Here's how the part is built. I have some questions about the finished solid (model axes, mm). Face numbers are marked on the shaded views. A direction names the side the tool comes from. Coordinates: 2 decimals unless noted, no trailing zeros. Write each loop counter-clockwise with the first axis right and the second up, starting at its lowest first coordinate (ties: lowest second). Pieces come first, ordered by that corner, then holes. Notation, with made-up numbers: (35, 42.5) - (67, 42.5) arc R13 ccw to (67, 65.5) - close; hole circle Ø10 at (20, 50). An arc over 180 degrees is marked (long way). Answer in a Markdown table with one row per item. Add a question column.
Item 1: Imagine slicing it at A-A (z = 0). Please give me the cut outline in (x, y), plus the area to 3 significant figures.
Item 2: I'm going to push flat-ended pins straight in: pin 1 (2 mm diameter, centred on x = -19.5, y = 17.5, fed in from -Z); pin 2 (12 mm diameter, centred on x = -7, z = -2.5, fed in from -Y); pin 3 (1.3 mm diameter, centred on x = 19, y = 21.5, fed in from -Z); pin 4 (6 mm diameter, centred on y = 133, z = -8.5, fed in from -X). Where does each tip first touch, or does it pass through?
Item 3: Imagine slicing it at D-D (x = 5). Please give me the cut outline in (y, z).
Item 4: Imagine slicing it at C-C (x = 14). Please give me the cut outline in (y, z).
Item 5: Which directions (+Z, -Z, +X, -X, +Y, -Y) give clear straight access to the entire face, cutting with the end or side of a thin tool? Please do the marked faces 1 and 2.
Item 6: If I drill on probe 1 along Y at (x, z) = (-7.5, 18.5); probe 2 along Y at (x, z) = (10, 18.5); probe 3 along Z at (x, y) = (10.5, 120), over which ranges is the centre line in solid material (lowest first)? Write a range as from..to.
Item 7: Imagine slicing it at B-B (y = 13.5). Please give me the cut outline in (x, z).
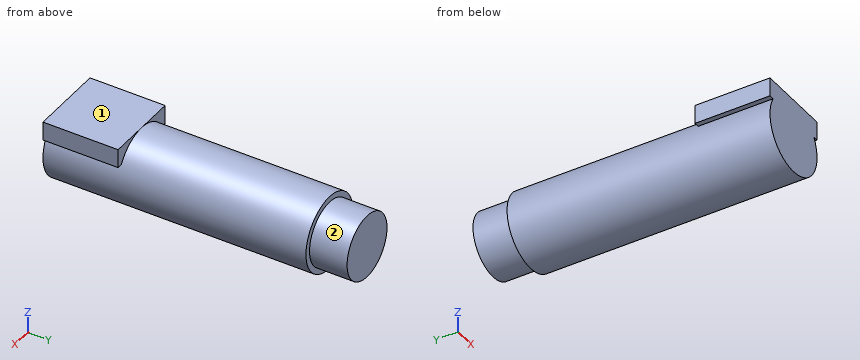
Autodesk Fusion 360 part; units mm, degrees
sketch "Sketch1" plane through (0, 0, 0) normal (0, 1, 0) x (1, 0, 0)
  circle A0 centre (0, 0) radius 20
  dimension "d1" = 40
extrude "Extrude1" add sketch "Sketch1" along normal blind 140
sketch "Sketch2" plane through (0, 140, 0) normal (0, 1, 0) x (-1, 0, 0)
  circle A0 centre (0, 0) radius 20
  circle A1 centre (0, 0) radius 17
  dimension "d4" = 34
extrude "Extrude2" add sketch "Sketch2" along normal blind 20 contours A1
sketch "Sketch3" plane through (0, 0, 0) normal (1, 0, 0) x (0, 0, -1)
sketch "Sketch4" plane through (0, 0, 0) normal (0, -1, 0) x (1, 0, 0)
  circle A0 centre (0, 0) radius 20
  line L0 (0, 20) -> (-20, 20)
  line L1 (-20, 20) -> (-20, 10)
  line L2 (-20, 10) -> (20, 10)
  line L3 (20, 10) -> (20, 20)
  line L4 (20, 20) -> (0, 20)
extrude "Extrude3" add sketch "Sketch4" against normal blind 40 contours A0 L2 L3 L4 | A0 L0 L1 L2
sketch "Sketch5" plane through (20, 0, 0) normal (1, 0, 0) x (0, 0, -1)
  line L0 (-20, 0) -> (-10, 0)
  line L1 (-10, 0) -> (-10, 40)
  line L2 (-10, 40) -> (-20, 40)
  line L3 (-20, 40) -> (-20, 0)
Here are the results:
| question | item | result |
|---|---|---|
| 1 | outline | (-20, 0) - (20, 0) - (20, 140) - (17, 140) - (17, 160) - (-17, 160) - (-17, 140) - (-20, 140) - close |
| 1 | area | 6,280 mm2 |
| 2 | pin 1 | stops at z = -7.6 |
| 2 | pin 2 | stops at y = 0 |
| 2 | pin 3 | stops at z = -7.95 |
| 2 | pin 4 | stops at x = -19.23 |
| 3 | outline | (0, -19.36) - (140, -19.36) - (140, -16.25) - (160, -16.25) - (160, 16.25) - (140, 16.25) - (140, 19.36) - (40, 19.36) - (40, 20) - (0, 20) - close |
| 4 | outline | (0, -14.28) - (140, -14.28) - (140, -9.64) - (160, -9.64) - (160, 9.64) - (140, 9.64) - (140, 14.28) - (40, 14.28) - (40, 20) - (0, 20) - close |
| 5 | face 1 | +Z, +X, -X, +Y, -Y |
| 5 | face 2 | +Y |
| 6 | probe 1 | y = 0..140 |
| 6 | probe 2 | y = 0..40 |
| 6 | probe 3 | z = -17.02..17.02 |
| 7 | outline | (-20, 10) - (-17.32, 10) arc R20 ccw (long way) to (17.32, 10) - (20, 10) - (20, 20) - (-20, 20) - close |
